Source: CAD feature listing. Evaluate the final solid. Frame: model axes, mm. Face numbers are marked on the shaded views. Coordinates: 2 decimals unless noted, no trailing zeros. Order: outer loops, then holes, each group sorted by start corner. A loop starts at its lowest first (then second) coordinate and runs counter-clockwise, first axis right, second up.
```python
from build123d import *

# Parameters (mm, degrees)
SKETCH1_W           = 55
SKETCH1_H           = 12
SKETCH1_R           = 2.98
BOSS_EXTRUDE1_DEPTH = 20
FILLET2_R           = 6


with BuildPart() as part:
    # Sketch1 → Boss-Extrude1 (new, symmetric)
    with BuildSketch(Plane.XY):
        with Locations((21.5, 0)):
            Rectangle(SKETCH1_W, SKETCH1_H)
        Circle(SKETCH1_R, mode=Mode.SUBTRACT)
    extrude(amount=BOSS_EXTRUDE1_DEPTH, both=True)

    # Fillet2
    fillet2_edges = [part.edges().sort_by_distance(p)[0] for p in [
        (49, -6, 0),
        (49, 6, 0),
        (-6, -6, 0),
        (-6, 6, 0),
    ]]
    fillet(fillet2_edges, radius=FILLET2_R - 0.0001)  # a hair under: the kernel refuses the full size


solid = part.part
```
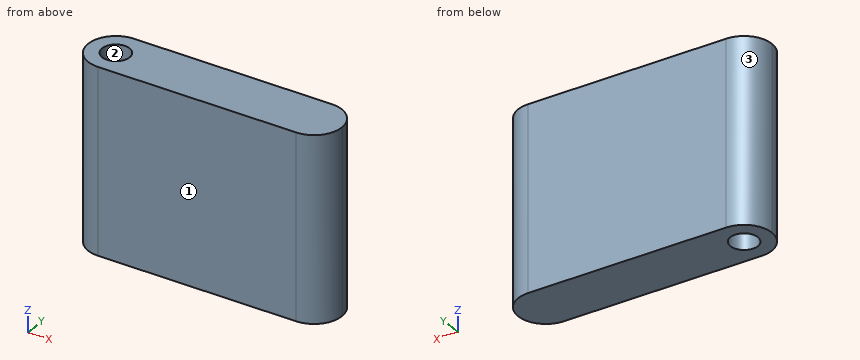
Q1. Pull-direction query (X, two-part tool) for the marked faces 1, 2 and 3; classes: pulls with the +X half, pulls with the -X half, needs draft (parallel to the pull), parting line crosses it, or undercut.
Solutions:
face 1: needs draft
face 2: undercut
face 3: pulls with the -X half
Q2. Material intervals for line 1 along Y through (x, z) = (0, -5.5); line 2 along X through (y, z) = (-0.25, 17); line 3 along X through (y, z) = (2.75, 15.5), sorted ascending.
Solutions:
line 1: y = -6 to -2.98, 2.98 to 6
line 2: x = -5.99 to -2.97, 2.97 to 48.99
line 3: x = -5.33 to -1.15, 1.15 to 48.33
Q3. Section query D-D on y = -4.5. Output: boundary loops of the cut face in (x, z), plus the area to 3 significant figures.
Solutions:
outline: (-3.97, -20) - (46.97, -20) - (46.97, 20) - (-3.97, 20) - close
area: 2,040 mm2
Q4. Section query B-B on y = -2. Output: boundary loops of the cut face in (x, z).
Solutions:
outline: (-5.66, -20) - (-2.21, -20) - (-2.21, 20) - (-5.66, 20) - close; (2.21, -20) - (48.66, -20) - (48.66, 20) - (2.21, 20) - close
Q5. Section query C-C on y = 1.5. Output: boundary loops of the cut face in (x, z), plus the area to 3 significant figures.
Solutions:
outline: (-5.81, -20) - (-2.57, -20) - (-2.57, 20) - (-5.81, 20) - close; (2.57, -20) - (48.81, -20) - (48.81, 20) - (2.57, 20) - close
area: 1,980 mm2
Q6. Pin query (flat end, axial travel): P1, Ø3.5, axis at x = 0, y = 0, coming from the +Z side. Return the tip coordinate at first contact, or that it passes through.
Solutions:
P1: passes through
